Verification items for the finished model (mm, model axes). Face numbers are marked on the shaded views. Round coordinates to 2 decimals unless told otherwise and drop trailing zeros. Order: outer loops, then holes, each group sorted by start corner. A loop starts at its lowest first (then second) coordinate and runs counter-clockwise, first axis right, second up. Notation, with made-up numbers: M -2,-37 L 37,-37 A23 ccw 37,-23 Z; hole C 84.5,-5 d2. An arc over 180 degrees is marked long. Answer as a JSON object with one key per item and string values. Group by question number.
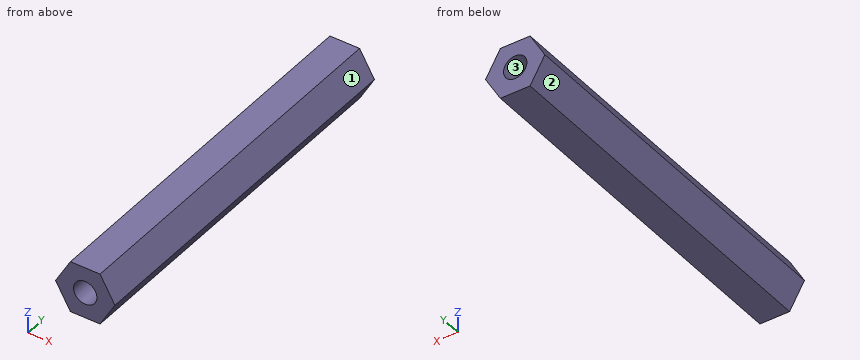
```python
from build123d import *

# Parameters (mm, degrees)
BOSS_EXTRUDE1_DEPTH = 20
M3_TAPPED_HOLE1_D   = 2.5


with BuildPart() as part:
    # Sketch1 → Boss-Extrude1 (new body, symmetric)
    with BuildSketch(Plane(origin=(0, 0, 0), x_dir=(1, 0, 0), z_dir=(0, 1, 0))):
        Polygon((3.175426481, 0), (1.58771324, 2.75), (-1.58771324, 2.75), (-3.175426481, 0), (-1.58771324, -2.75), (1.58771324, -2.75), align=None)
    extrude(amount=BOSS_EXTRUDE1_DEPTH, both=True)

    # M3 Tapped Hole1 (through all)
    with Locations(Plane(origin=(0, 20, 0), x_dir=(1, 0, 0), z_dir=(0, 1, 0))):
        with Locations((0, 0)):
            Hole(M3_TAPPED_HOLE1_D / 2)


solid = part.part
```
Q1. Cross-section at B-B, the plane x = 0. Record the cut outline in (y, z).
Q2. Gauge pin test, flat ends, axial feed: pin 1 Ø2 at (y, z) = (-0.5, 2) entering from +X; pin 2 Ø1.5 at (y, z) = (9.5, 1.5) entering from -X. Record the tip position at first contact, or that the pin passes through.
Q3. Cross-section at A-A, the plane y = 17. Record the cut outline in (x, z), then the cut area to 3 significant figures.
Q4. Cross-section at C-C, the plane z = 0.65. Record the cut outline in (x, y), then the cut area to 3 significant figures.
Q5. Release check for a two-part mould opening along Z. For the marked faces 1, 2 and 3 record: released by +Z, released by -Z, zero draft, split by the parting line, or undercut.
Q6. Thickness scan on line 1 (Z direction, x = 0, y = -4.5); line 2 (X direction, y = -6, z = -0.55); line 3 (Z direction, x = -1, y = -4). Record the ranges inside material, lowest first. Write a range as from..to.
Q7. Cross-section at D-D, the plane x = -2.5. Record the cut outline in (y, z), then the cut area to 3 significant figures.
Conclusion:
{
 "1": {"outline": "M -20,-2.75 L 20,-2.75 L 20,-1.25 L -20,-1.25 Z; M -20,1.25 L 20,1.25 L 20,2.75 L -20,2.75 Z"},
 "2": {"pin 1": "x = 2.6", "pin 2": "x = -2.74"},
 "3": {"outline": "M -3.18,0 L -1.59,-2.75 L 1.59,-2.75 L 3.18,0 L 1.59,2.75 L -1.59,2.75 Z; hole C 0,0 d2.5", "area": "21.3 mm2"},
 "4": {"outline": "M -2.8,-20 L -1.07,-20 L -1.07,20 L -2.8,20 Z; M 1.07,-20 L 2.8,-20 L 2.8,20 L 1.07,20 Z", "area": "139 mm2"},
 "5": {"face 1": "released by +Z", "face 2": "released by -Z", "face 3": "undercut"},
 "6": {"line 1": "-2.75..-1.25, 1.25..2.75", "line 2": "-2.86..-1.12, 1.12..2.86", "line 3": "-2.75..-0.75, 0.75..2.75"},
 "7": {"outline": "M -20,-1.17 L 20,-1.17 L 20,1.17 L -20,1.17 Z", "area": "93.6 mm2"}
}
